The listing builds one solid part. Answer for the finished solid, in the listing's coordinates (mm). A direction names the side the tool comes from. Give positions to 0.01 mm unless a question says otherwise; leave off trailing zeros. Write each loop counter-clockwise with the first axis right and the second up, starting at its lowest first coordinate (ties: lowest second). Pieces come first, ordered by that corner, then holes. Notation, with made-up numbers: (50, 39) - (82, 39) arc R24 ccw to (82, 65) - close; hole circle Ø9 at (13, 32.5). An arc over 180 degrees is marked (long way). Answer as CSV lines item,"result". Start each with the question number.
(1) Straight lines are drawn through the part: probe 1 along Z at (x, y) = (-59.5, 19); probe 2 along Y at (x, z) = (-63.6, -19); probe 3 along X at (y, z) = (7.5, -12). For each, find the intervals that lie inside material, in ascending order.
(2) For faces 5 (the face through (-30, 25, -29.5)), 6 (the face through (0, 43, 64)), 7 (the face through (0, 47, 60.5)), determine the directions among +Z, -Z, +X, -X, +Y, -Y from which every point of the face is accessible in a straight line to the end or side of a thin tool.
(3) Each of these flat-tipped pins is pushed along its axis until it touches: pin 1 Ø13 at (y, z) = (32, -19) entering from +X; pin 2 Ø1.5 at (x, z) = (-23.5, 41) entering from +Y. Where does it stop, or does it pass through?
(4) Find section C-C (x = -57). Write down the section's boundary in (y, z).
(5) Find section D-D (z = 51). Write down the section's boundary in (x, y).
(6) Find section B-B (y = 32). Write down the section's boundary in (x, z).
(7) Find section A-A (y = 6.5). Write down the section's boundary in (x, z), then the cut area to 3 significant figures.
(8) For a pull along X with two mould halves and no side action, classify faces 1 (the face through (-64.696, 25, 21)), 2 (the face through (0, 47, -19.5)), 3 (the face through (6.304, 25, 21)), 4 (the face through (-58, 47, -19.5)) as pulls with the +X half, pulls with the -X half, needs draft (parallel to the pull), parting line crosses it, or undercut.
from build123d import *

# Parameters (mm, degrees)
SKETCH1_W               = 71
SKETCH1_H               = 100
BOSS_EXTRUDE1_DEPTH     = 50
SKETCH2_W               = 65
SKETCH2_H               = 94
CUT_EXTRUDE1_DEPTH      = 47
SKETCH3_W               = 51
SKETCH3_H               = 61.662084765
BOSS_EXTRUDE2_DEPTH     = 5
CUT_EXTRUDE2_DEPTH      = 110.973860531
CUT_EXTRUDE2_DEPTH_BACK = 110.973860531
SKETCH4_R               = 5
SKETCH5_W               = 10
SKETCH5_H               = 10
SKETCH5_W_2             = 9.971264926
BOSS_EXTRUDE3_DEPTH     = 7


with BuildPart() as part:
    # Sketch1 → Boss-Extrude1 (new body)
    with BuildSketch(Plane(origin=(0, 0, 0), x_dir=(1, 0, 0), z_dir=(0, 1, 0))):
        with Locations((-29.196168954, -20.5)):
            Rectangle(SKETCH1_W, SKETCH1_H)
    extrude(amount=BOSS_EXTRUDE1_DEPTH)

    # Sketch2 → Cut-Extrude1 (cut)
    with BuildSketch(Plane(origin=(0, 50, 0), x_dir=(1, 0, 0), z_dir=(0, 1, 0))):
        with Locations((-29.196168954, -20.5)):
            Rectangle(SKETCH2_W, SKETCH2_H)
    extrude(amount=-CUT_EXTRUDE1_DEPTH, mode=Mode.SUBTRACT)

    # Sketch3 → Boss-Extrude2 (add)
    with BuildSketch(Plane(origin=(0, 3, 0), x_dir=(1, 0, 0), z_dir=(0, 1, 0))):
        with Locations((-36.196168954, -4.331042383)):
            Rectangle(SKETCH3_W, SKETCH3_H)
    extrude(amount=BOSS_EXTRUDE2_DEPTH)

    # Sketch4 → Cut-Extrude2 (cut, two sides: drawn at the far end of the back side and taken through both)
    with BuildSketch(Plane(origin=(-61.696168954, 0, 0), x_dir=(0, 0, -1), z_dir=(1, 0, 0)).offset(-CUT_EXTRUDE2_DEPTH_BACK)):
        with Locations((19, 32)):
            Circle(SKETCH4_R)
    extrude(amount=CUT_EXTRUDE2_DEPTH + CUT_EXTRUDE2_DEPTH_BACK, mode=Mode.SUBTRACT)

    # Sketch5 → Boss-Extrude3 (add)
    with BuildSketch(Plane(origin=(0, 50, 0), x_dir=(1, 0, 0), z_dir=(0, 1, 0))):
        with Locations((-59.696168954, 24.5)):
            Rectangle(SKETCH5_W, SKETCH5_H)
        with Locations((1.318198583, 24.5)):
            Rectangle(SKETCH5_W_2, SKETCH5_H)
        with Locations((1.303831046, -65.5)):
            Rectangle(SKETCH5_W, SKETCH5_H)
        with Locations((-59.696168954, -65.5)):
            Rectangle(SKETCH5_W, SKETCH5_H)
    extrude(amount=-BOSS_EXTRUDE3_DEPTH)


solid = part.part
Result set:
1,probe 1,"-29.5 to -26.5, 67.5 to 70.5"
1,probe 2,"0 to 27, 37 to 50"
1,probe 3,"-64.7 to -10.7, 3.3 to 6.3"
2,face 5,"-Z, +X, -X, +Y, -Y"
2,face 6,"none"
2,face 7,"+Y"
3,pin 1,"x = 6.3"
3,pin 2,"y = 3"
4,outline,"(0, -29.5) - (50, -29.5) - (50, -19.5) - (43, -19.5) - (43, -26.5) - (8, -26.5) - (8, 35.16) - (3, 35.16) - (3, 67.5) - (43, 67.5) - (43, 60.5) - (50, 60.5) - (50, 70.5) - (0, 70.5) - close"
5,outline,"(-64.7, 0) - (6.3, 0) - (6.3, 50) - (3.3, 50) - (3.3, 3) - (-61.7, 3) - (-61.7, 50) - (-64.7, 50) - close"
6,outline,"(-64.7, -29.5) - (6.3, -29.5) - (6.3, -24) - (3.3, -24) - (3.3, -26.5) - (-61.7, -26.5) - (-61.7, -24) - (-64.7, -24) - close; (-64.7, -14) - (-61.7, -14) - (-61.7, 67.5) - (3.3, 67.5) - (3.3, -14) - (6.3, -14) - (6.3, 70.5) - (-64.7, 70.5) - close"
7,outline,"(-64.7, -29.5) - (6.3, -29.5) - (6.3, 70.5) - (-64.7, 70.5) - close; hole (-61.7, 35.16) - (-10.7, 35.16) - (-10.7, -26.5) - (3.3, -26.5) - (3.3, 67.5) - (-61.7, 67.5) - close"
7,area,"4,130 mm^2"
8,face 1,"pulls with the -X half"
8,face 2,"undercut"
8,face 3,"pulls with the +X half"
8,face 4,"undercut"
